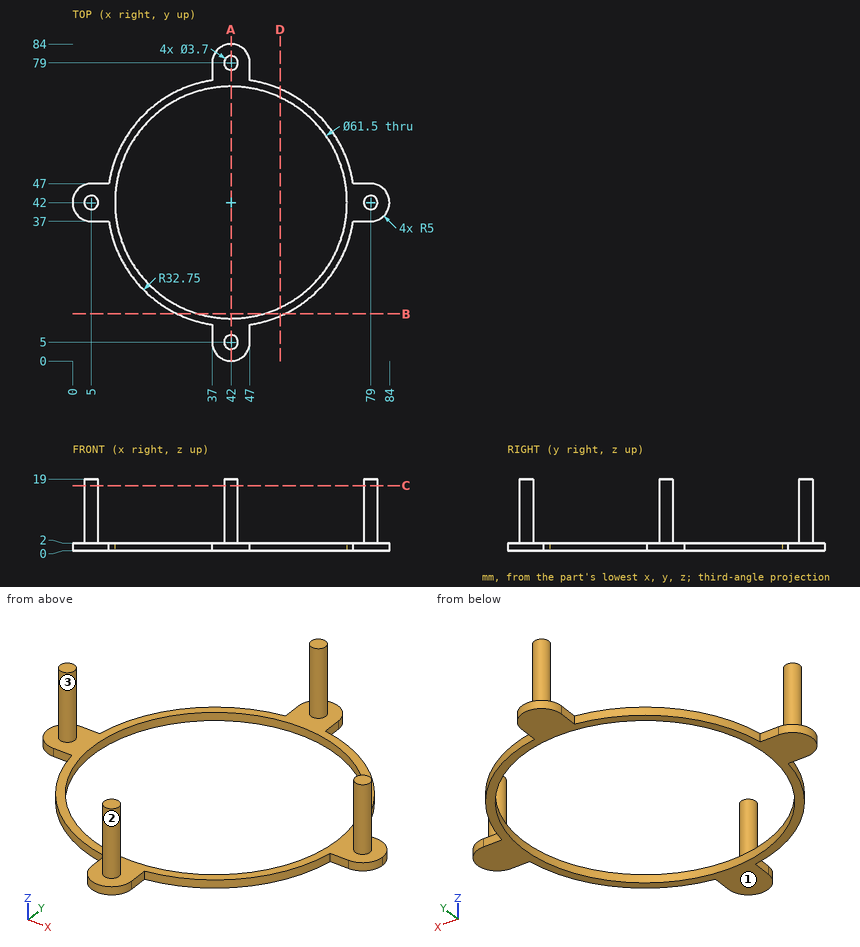
Design review of the part shown in the three views and the two pictorial views. Dimensions are in mm from the part's minimum x, y and z. Round coordinates to 2 decimals unless told otherwise and drop trailing zeros. Loops run counter-clockwise (first coordinate to the right, second up) from the corner with the lowest first, then second, coordinate; pieces in that order, holes last. Notation, with made-up numbers: (-1, -7) -> (25, -7) arc R20 cw to (25, 16) -> close; hole circle Ø8 at (9, -34.75). An arc over 180 degrees is marked (long way). Answer as a JSON object with one key per item and string values. Group by question number.
1) We need section C-C on z = 17.25. Write out the cut boundary in (x, y), then the cut area to 3 significant figures.
2) We need section D-D on x = 55. Write out the cut boundary in (y, z).
3) For line 1 (Y direction, x = 42, z = 0.65); line 2 (Z direction, x = 58, y = 14); line 3 (X direction, y = 6, z = 15.25), list the stretches that pass through material, from the lowest coordinate up. Write a range as [from, to].
4) Mouldability with a two-part tool opening along Y and no side actions: class the marked faces 1, 2 and 3 as released by +Y, released by -Y, zero draft, split by the parting line, or undercut.
5) For pin 1 Ø6 at (x, z) = (40.5, 7) entering from +Y; pin 2 Ø1 at (x, z) = (76.5, 1) entering from +Y; pin 3 Ø1 at (y, z) = (75.5, 1) entering from +X; pin 4 Ø8 at (x, z) = (44.5, 3) entering from +Y, all flat-tipped, find the tip position at first contact; note any pin that passes through.
6) We need section B-B on y = 12.5. Write out the cut boundary in (x, z).
7) We need section A-A on x = 42. Write out the cut boundary in (y, z), then the cut area to 3 significant figures.
Result set:
{
 "1": {"outline": "circle Ø3.7 at (5, 42); circle Ø3.7 at (42, 5); circle Ø3.7 at (42, 79); circle Ø3.7 at (79, 42)", "area": "43.0 mm²"},
 "2": {"outline": "(11.94, 0) -> (14.13, 0) -> (14.13, 2) -> (11.94, 2) -> close; (69.87, 0) -> (72.06, 0) -> (72.06, 2) -> (69.87, 2) -> close"},
 "3": {"line 1": "[0, 11.25], [72.75, 84]", "line 2": "[0, 2]", "line 3": "[40.44, 43.56]"},
 "4": {"face 1": "zero draft", "face 2": "undercut", "face 3": "split by the parting line"},
 "5": {"pin 1": "y = 80.85", "pin 2": "y = 47", "pin 3": "x = 47", "pin 4": "y = 84"},
 "6": {"outline": "(27.78, 0) -> (33.32, 0) -> (33.32, 2) -> (27.78, 2) -> close; (50.68, 0) -> (56.22, 0) -> (56.22, 2) -> (50.68, 2) -> close"},
 "7": {"outline": "(0, 0) -> (11.25, 0) -> (11.25, 2) -> (6.85, 2) -> (6.85, 19) -> (3.15, 19) -> (3.15, 2) -> (0, 2) -> close; (72.75, 0) -> (84, 0) -> (84, 2) -> (80.85, 2) -> (80.85, 19) -> (77.15, 19) -> (77.15, 2) -> (72.75, 2) -> close", "area": "171 mm²"}
}
